Autodesk Inventor part; units mm, degrees
ref_plane "YZ Plane" through (0, 0, 0) normal (1, 0, 0) x (0, 1, 0)
ref_plane "XZ Plane" through (0, 0, 0) normal (0, 1, 0) x (-1, 0, 0)
ref_plane "XY Plane" through (0, 0, 0) normal (0, 0, 1) x (1, 0, 0)
sketch "スケッチ1" plane through (0, 0, 0) normal (0, 0, 1) x (1, 0, 0)
  line L0 (-25.3, 21.7) -> (25.3, 21.7)
  line L1 (25.3, 21.7) -> (25.3, -21.7)
  line L2 (25.3, -21.7) -> (-25.3, -21.7)
  line L3 (-25.3, -21.7) -> (-25.3, 21.7)
  circle A0 centre (-22.1, 18.5) radius 1.3
  circle A1 centre (22.1, 18.5) radius 1.3
  circle A2 centre (22.1, -18.5) radius 1.3
  circle A3 centre (-22.1, -18.5) radius 1.3
  line L4 (-18.1, 19.2) -> (-18.1, 14.5)
  line L5 (-18.1, 14.5) -> (-22.8, 14.5)
  line L6 (-22.8, 14.5) -> (-22.8, -14.5)
  line L7 (-22.8, -14.5) -> (-18.1, -14.5)
  line L8 (-18.1, -14.5) -> (-18.1, -19.2)
  line L9 (-18.1, -19.2) -> (18.1, -19.2)
  line L10 (18.1, -19.2) -> (18.1, -14.5)
  line L11 (18.1, -14.5) -> (22.8, -14.5)
  line L12 (22.8, -14.5) -> (22.8, 14.5)
  line L13 (22.8, 14.5) -> (18.1, 14.5)
  line L14 (18.1, 14.5) -> (18.1, 19.2)
  line L15 (18.1, 19.2) -> (-18.1, 19.2)
  point P0 (0, 0)
  point P1 (0, 21.7)
  point P2 (-25.3, 0)
  dimension "d0" = 50.6
  dimension "d1" = 43.4
  dimension "d2" = 2.6
  dimension "d3" = 44.2
  dimension "d4" = 37
  dimension "d5" = 22.1
  dimension "d6" = 18.5
  dimension "d7" = 2.5
  dimension "d8" = 2.5
  dimension "d9" = 2.5
  dimension "d10" = 2.5
  dimension "d11" = 4
  dimension "d12" = 4
  dimension "d13" = 4
  dimension "d14" = 4
  dimension "d15" = 4
extrude "押し出し1" add sketch "スケッチ1" along normal blind 6.9
sketch "スケッチ4" plane through (0, 0, 6.9) normal (0, 0, 1) x (1, 0, 0)
  line L0 (-18.1, 14.5) -> (-18.1, 19.2)
  line L1 (-18.1, 19.2) -> (18.1, 19.2)
  line L2 (-22.8, 14.5) -> (-18.1, 14.5)
  line L3 (-22.8, -14.5) -> (-22.8, 14.5)
  line L4 (-18.1, -14.5) -> (-22.8, -14.5)
  line L5 (-18.1, -19.2) -> (-18.1, -14.5)
  line L6 (18.1, -19.2) -> (-18.1, -19.2)
  line L7 (18.1, -14.5) -> (18.1, -19.2)
  line L8 (22.8, -14.5) -> (18.1, -14.5)
  line L9 (22.8, 14.5) -> (22.8, -14.5)
  line L10 (18.1, 14.5) -> (22.8, 14.5)
  line L11 (18.1, 19.2) -> (18.1, 14.5)
  point P0 (0, 0)
extrude "押し出し4" add sketch "スケッチ4" against normal blind 3
sketch "スケッチ3" plane through (0, 0, 6.9) normal (0, 0, 1) x (1, 0, 0)
  line L0 (-14.6, 19.9) -> (-3.9, 19.9) construction
  line L1 (-3.9, 19.9) -> (-3.9, 13.6) construction
  line L2 (-3.9, 13.6) -> (-14.6, 13.6) construction
  line L3 (-14.6, 13.6) -> (-14.6, 19.9) construction
  line L4 (-1.6, 19.9) -> (9.1, 19.9) construction
  line L5 (9.1, 19.9) -> (9.1, 13.6) construction
  line L6 (9.1, 13.6) -> (-1.6, 13.6) construction
  line L7 (-1.6, 13.6) -> (-1.6, 19.9) construction
  line L8 (13, 19.8) -> (19.3, 19.8) construction
  line L9 (19.3, 19.8) -> (19.3, 9.1) construction
  line L10 (19.3, 9.1) -> (13, 9.1) construction
  line L11 (13, 9.1) -> (13, 19.8) construction
  line L12 (25.3, 21.7) -> (-25.3, 21.7) construction
  line L13 (25.3, -21.7) -> (25.3, 21.7) construction
  line L14 (-14.8, 13.4) -> (-3.7, 13.4)
  line L15 (-3.7, 13.4) -> (-3.7, 20.1)
  line L16 (-3.7, 20.1) -> (-14.8, 20.1)
  line L17 (-14.8, 20.1) -> (-14.8, 13.4)
  line L18 (-1.8, 13.4) -> (9.3, 13.4)
  line L19 (9.3, 13.4) -> (9.3, 20.1)
  line L20 (9.3, 20.1) -> (-1.8, 20.1)
  line L21 (-1.8, 20.1) -> (-1.8, 13.4)
  line L22 (12.8, 8.9) -> (19.5, 8.9)
  line L23 (19.5, 8.9) -> (19.5, 20)
  line L24 (19.5, 20) -> (12.8, 20)
  line L25 (12.8, 20) -> (12.8, 8.9)
  point P0 (0, 0)
  dimension "d20" = 6.3
  dimension "d21" = 10.7
  dimension "d23" = 6
  dimension "d24" = 1.8
  dimension "d25" = 26.9
  dimension "d26" = 39.9
  dimension "d27" = 12.6
  dimension "d28" = 0.2
  dimension "d29" = 0.2
  dimension "d30" = 0.2
extrude "押し出し3" cut sketch "スケッチ3" along normal through all both and the other way through all
sketch "スケッチ5" plane through (0, 0, 6.9) normal (0, 0, 1) x (1, 0, 0)
  line L0 (-21.5, 13.3) -> (-13.8, 13.3) construction
  line L1 (-13.8, 13.3) -> (-13.8, 3.3) construction
  line L2 (-13.8, 3.3) -> (-21.5, 3.3) construction
  line L3 (-21.5, 3.3) -> (-21.5, 13.3) construction
  line L4 (25.3, 21.7) -> (-25.3, 21.7) construction
  line L5 (25.3, -21.7) -> (25.3, 21.7) construction
  line L6 (-25.3, 13.5) -> (-13.6, 13.5)
  line L7 (-13.6, 13.5) -> (-13.6, 3.1)
  line L8 (-13.6, 3.1) -> (-25.3, 3.1)
  line L9 (-25.3, 3.1) -> (-25.3, 13.5)
  line L10 (-25.3, 21.7) -> (-25.3, -21.7) construction
  point P0 (0, 0)
  dimension "d35" = 46.8
  dimension "d36" = 7.7
  dimension "d37" = 18.4
  dimension "d38" = 10
  dimension "d39" = 0.2
  dimension "d40" = 0.2
  dimension "d41" = 0.2
extrude "押し出し5" cut sketch "スケッチ5" against normal through all
sketch "スケッチ6" plane through (0, 0, 6.9) normal (0, 0, 1) x (1, 0, 0)
  line L0 (-5.2, 2.3) -> (-15, 2.3) construction
  line L1 (-15, 2.3) -> (-15, -11.9) construction
  line L2 (-15, -11.9) -> (-5.2, -11.9) construction
  line L3 (-5.2, -11.9) -> (-5.2, 2.3) construction
  line L4 (25.3, 21.7) -> (-25.3, 21.7) construction
  line L5 (25.3, -21.7) -> (25.3, 21.7) construction
  line L6 (-15.2, 2.5) -> (-5, 2.5)
  line L7 (-5, 2.5) -> (-5, -12.1)
  line L8 (-5, -12.1) -> (-15.2, -12.1)
  line L9 (-15.2, -12.1) -> (-15.2, 2.5)
  point P0 (0, 0)
  dimension "d44" = 14.2
  dimension "d45" = 9.8
  dimension "d46" = 40.3
  dimension "d47" = 33.6
  dimension "d48" = 0.2
extrude "押し出し6" cut sketch "スケッチ6" against normal through all
sketch "スケッチ7" plane through (0, 0, 6.9) normal (0, 0, 1) x (1, 0, 0)
  line L0 (25.3, 21.7) -> (-25.3, 21.7) construction
  line L1 (25.3, -21.7) -> (25.3, 21.7) construction
  line L2 (12.8, -5.3) -> (18.6, -5.3) construction
  line L3 (18.6, -5.3) -> (18.6, -12.8) construction
  line L4 (18.6, -12.8) -> (12.8, -12.8) construction
  line L5 (12.8, -12.8) -> (12.8, -5.3) construction
  line L6 (-9.5, -14.8) -> (-2, -14.8) construction
  line L7 (-2, -14.8) -> (-2, -20.6) construction
  line L8 (-2, -20.6) -> (-9.5, -20.6) construction
  line L9 (-9.5, -20.6) -> (-9.5, -14.8) construction
  line L10 (12.6, -13) -> (18.8, -13)
  line L11 (18.8, -13) -> (18.8, -5.1)
  line L12 (18.8, -5.1) -> (12.6, -5.1)
  line L13 (12.6, -5.1) -> (12.6, -13)
  line L14 (-1.8, -20.8) -> (-1.8, -14.6)
  line L15 (-1.8, -14.6) -> (-9.7, -14.6)
  line L16 (-9.7, -14.6) -> (-9.7, -20.8)
  line L17 (-9.7, -20.8) -> (-1.8, -20.8)
  point P0 (0, 0)
  dimension "d51" = 7.5
  dimension "d52" = 5.8
  dimension "d53" = 12.5
  dimension "d54" = 34.5
  dimension "d55" = 42.3
  dimension "d56" = 34.8
  dimension "d57" = 0.2
  dimension "d58" = 0.2
extrude "押し出し7" cut sketch "スケッチ7" against normal through all
sketch "スケッチ8" plane through (0, 0, 6.9) normal (0, 0, 1) x (1, 0, 0)
  circle A0 centre (-18, -0.6) radius 2.5 construction
  circle A1 centre (-12.5, -14.6) radius 2.5 construction
  line L0 (25.3, 21.7) -> (-25.3, 21.7) construction
  line L1 (25.3, -21.7) -> (25.3, 21.7) construction
  circle A2 centre (-18, -0.6) radius 2.7
  circle A3 centre (-12.5, -14.6) radius 2.7
  point P0 (0, 0)
  dimension "d61" = 5
  dimension "d62" = 22.3
  dimension "d63" = 36.3
  dimension "d64" = 43.3
  dimension "d65" = 37.8
  dimension "d66" = 0.2
  dimension "d67" = 0.2
extrude "押し出し8" cut sketch "スケッチ8" against normal through all
sketch "スケッチ9" plane through (0, 0, 6.9) normal (0, 0, 1) x (1, 0, 0)
  line L0 (11.3, 1.5) -> (11.3, 7.3) construction
  line L1 (11.3, 7.3) -> (17.8, 7.3) construction
  line L2 (17.8, 7.3) -> (17.8, 1.5) construction
  line L3 (17.8, 1.5) -> (16.3, 0) construction
  line L4 (16.3, 0) -> (12.8, 0) construction
  line L5 (12.8, 0) -> (11.3, 1.5) construction
  line L6 (-0.7, 1.5) -> (-0.7, 7.3) construction
  line L7 (-0.7, 7.3) -> (5.8, 7.3) construction
  line L8 (5.8, 7.3) -> (5.8, 1.5) construction
  line L9 (5.8, 1.5) -> (4.3, 0) construction
  line L10 (4.3, 0) -> (0.8, 0) construction
  line L11 (0.8, 0) -> (-0.7, 1.5) construction
  line L12 (25.3, -21.7) -> (25.3, 21.7) construction
  line L13 (25.3, 21.7) -> (-25.3, 21.7) construction
  line L14 (6, 7.5) -> (-0.9, 7.5)
  line L15 (-0.9, 7.5) -> (-0.9, 1.4172)
  line L16 (-0.9, 1.4172) -> (0.7172, -0.2)
  line L17 (0.7172, -0.2) -> (4.3828, -0.2)
  line L18 (4.3828, -0.2) -> (6, 1.4172)
  line L19 (6, 1.4172) -> (6, 7.5)
  line L20 (18, 7.5) -> (11.1, 7.5)
  line L21 (11.1, 7.5) -> (11.1, 1.4172)
  line L22 (11.1, 1.4172) -> (12.7172, -0.2)
  line L23 (12.7172, -0.2) -> (16.3828, -0.2)
  line L24 (16.3828, -0.2) -> (18, 1.4172)
  line L25 (18, 1.4172) -> (18, 7.5)
  point P0 (0, 0)
  dimension "d70" = 135
  dimension "d71" = 135
  dimension "d72" = 135
  dimension "d73" = 135
  dimension "d74" = 7.3
  dimension "d75" = 6.5
  dimension "d76" = 1.5
  dimension "d77" = 26
  dimension "d78" = 14
  dimension "d79" = 21.7
  dimension "d80" = 0.2
  dimension "d81" = 0.2
extrude "押し出し9" cut sketch "スケッチ9" against normal through all
sketch "スケッチ10" plane through (0, 0, 6.9) normal (0, 0, 1) x (1, 0, 0)
  arc A0 (-13.5198, -12.1) -> (-11.4802, -12.1) centre (-12.5, -14.6) ccw construction
  circle A1 centre (-18, -0.6) radius 2.7 construction
  line L0 (-13.6, 13.4) -> (-13.6, 3.1) construction
  line L1 (-15.2, -12.1) -> (-15.2, 2.5) construction
  line L2 (-9.7, -14.6) -> (-1.8, -14.6) construction
  line L3 (-12.5, -14.6) -> (-15.2, -14.6) construction
  line L4 (-5, -14.6881) -> (-5, -8.3419)
  line L5 (-5, -8.3419) -> (-15.2, -8.3419)
  line L6 (-15.2, -8.3419) -> (-15.2, -14.6)
  line L7 (-15.2, -14.6) -> (-12.5, -14.6)
  line L8 (-12.5, -14.6) -> (-12.5, -17.3)
  line L9 (-12.5, -17.3) -> (-5, -17.3)
  line L10 (-5, -17.3) -> (-5, -14.6881)
  line L11 (-9.7, -20.8) -> (-9.7, -14.6) construction
  line L12 (-20.7, 3.1) -> (-20.7, -0.6)
  line L13 (-20.7, -0.6) -> (-18, -0.6)
  line L14 (-18, -0.6) -> (-18, -3.3)
  line L15 (-18, -3.3) -> (-13.6, -3.3)
  line L16 (-13.6, -3.3) -> (-13.6, 3.1)
  line L17 (-13.6, 3.1) -> (-20.7, 3.1)
  point P0 (0, 0)
  point P1 (-5, -12.1)
extrude "押し出し10" cut sketch "スケッチ10" against normal through all
sketch "スケッチ11" plane through (-25.3, 21.7, 0) normal (0, 1, 0) x (1, 0, 0)
  line L0 (50.6, -6.9) -> (0, -6.9)
  line L1 (50.6, 0) -> (50.6, -6.9)
  line L2 (50.6, 0) -> (0, 0)
  line L3 (0, 0) -> (0, -6.9)
  point P0 (25.3, 0)
extrude "押し出し11" add sketch "スケッチ11" along normal blind 3.6
sketch "スケッチ12" plane through (-25.3, -21.7, 0) normal (0, -1, 0) x (1, 0, 0)
  line L0 (0, 0) -> (0, 6.9)
  line L1 (0, 0) -> (50.6, 0)
  line L2 (0, 6.9) -> (50.6, 6.9)
  line L3 (50.6, 0) -> (50.6, 6.9)
  point P0 (25.3, 0)
extrude "押し出し12" add sketch "スケッチ12" along normal blind 3.6
sketch "スケッチ13" plane through (0, 0, 0) normal (0, 0, -1) x (-1, 0, 0)
  line L0 (-25.3, 25.3) -> (25.3, 25.3)
  line L1 (25.3, -25.3) -> (-25.3, -25.3)
  line L2 (-25.3, 21.9) -> (25.3, 21.9)
  line L3 (25.3, -21.9) -> (-25.3, -21.9)
  line L4 (25.3, 21.9) -> (25.3, 25.3)
  line L5 (-25.3, 25.3) -> (-25.3, 21.9)
  line L6 (25.3, -21.9) -> (25.3, -25.3)
  line L7 (-25.3, -21.9) -> (-25.3, -25.3)
  point P0 (0, 0)
  dimension "d90" = 3.4
  dimension "d91" = 3.4
extrude "押し出し13" add sketch "スケッチ13" along normal blind 1.6
equation "\"d8\" = d7"
equation "\"d9\" = d7"
equation "\"d10\" = d7"
equation "\"d12\" = d11"
equation "\"d13\" = d11"
equation "\"d14\" = d11"
equation "\"d15\" = d11"
equation "\"d40\" = d39"
equation "\"d41\" = d39"
equation "\"d71\" = d70"
equation "\"d73\" = d72"
equation "\"d81\" = d80"
properties part number "fan_controller_case_top"
Read the model definition and answer for the solid it produces. Units are mm, in the model's axes. A direction names the side the tool comes from. Round coordinates to 2 decimals unless told otherwise and drop trailing zeros. Write each loop counter-clockwise with the first axis right and the second up, starting at its lowest first coordinate (ties: lowest second). Pieces come first, ordered by that corner, then holes. Notation, with made-up numbers: M -9.75,82 L 4.25,82 A8 ccw 4.25,87 Z; hole C 35,44 d3. An arc over 180 degrees is marked long. Use a Markdown table: item, result.
1) The part is cut by section D-D (x = 22.1). Write down the section's boundary in (y, z).
Answers follow:
| item | result |
|---|---|
| outline | M -25.3,-1.6 L -21.9,-1.6 L -21.9,0 L -19.8,0 L -19.8,6.9 L -25.3,6.9 Z; M -17.2,0 L -14.5,0 L -14.5,3.9 L 14.5,3.9 L 14.5,0 L 17.2,0 L 17.2,6.9 L -17.2,6.9 Z; M 19.8,0 L 21.9,0 L 21.9,-1.6 L 25.3,-1.6 L 25.3,6.9 L 19.8,6.9 Z |
2) A tool of negligible diameter and unlimited length cuts with its end or side. For faces 1 (the flat face through (0, -21.9, -1)), 2 (the flat face through (0, 0, 6.9)), 3 (the flat face through (-15.2, -9, 5)), 4 (the flat face through (22.8, 0, 2)), from which of +Z, -Z, +X, -X, +Y, -Y can it reach the whole face along a straight path? Write none if from no direction.
Answers follow:
| item | result |
|---|---|
| face 1 | -Z, +X, -X |
| face 2 | +Z, +X, -X, +Y, -Y |
| face 3 | +Z, -Z |
| face 4 | -Z |
3) Flat-ended cylindrical pins translate along their axes: pin 1 (6 mm diameter, centred on x = 3.5, y = 3.5, fed in from +Z); pin 2 (6 mm diameter, centred on x = -10.5, y = 6.5, fed in from -Z); pin 3 (3.5 mm diameter, centred on y = 8.5, z = 6, fed in from -X); pin 4 (14.5 mm diameter, centred on x = -16, y = -9, fed in from -Z). Find the tip coordinate at first contact, or state that the pin passes through.
Answers follow:
| item | result |
|---|---|
| pin 1 | stops at z = 6.9 |
| pin 2 | stops at z = 3.9 |
| pin 3 | stops at x = -13.6 |
| pin 4 | stops at z = 0 |
4) Straight lines are drawn through the part: line 1 along X through (y, z) = (6, 4); line 2 along Y through (x, z) = (-22.1, 4.25); line 3 along Y through (x, z) = (22.1, 5.25). For each, find the intervals that lie inside material, in ascending order. Write a range as [from, to].
Answers follow:
| item | result |
|---|---|
| line 1 | x = [-13.6, -0.9], [6, 11.1], [18, 25.3] |
| line 2 | y = [-25.3, -19.8], [-17.2, 3.1], [13.5, 17.2], [19.8, 25.3] |
| line 3 | y = [-25.3, -19.8], [-17.2, 17.2], [19.8, 25.3] |
5) The part is cut by section B-B (y = -18.5). Write down the section's boundary in (x, z), plus the area to 3 significant figures.
Answers follow:
| item | result |
|---|---|
| outline | M -25.3,0 L -23.4,0 L -23.4,6.9 L -25.3,6.9 Z; M -20.8,0 L -18.1,0 L -18.1,3.9 L -9.7,3.9 L -9.7,6.9 L -20.8,6.9 Z; M -1.8,3.9 L 18.1,3.9 L 18.1,0 L 20.8,0 L 20.8,6.9 L -1.8,6.9 Z; M 23.4,0 L 25.3,0 L 25.3,6.9 L 23.4,6.9 Z |
| area | 148 mm2 |
6) For a pull along X with two mould halves and no side action, classify faces 5 (the flat face through (3, 7.5, 5)), 6 (the flat face through (-0.1, -19.4, 0)), 7 (the flat face through (-25.3, -11, 4)) as pulls with the +X half, pulls with the -X half, needs draft (parallel to the pull), parting line crosses it, or undercut.
Answers follow:
| item | result |
|---|---|
| face 5 | undercut |
| face 6 | needs draft |
| face 7 | pulls with the -X half |
7) The part is cut by section C-C (y = 18.5). Write down the section's boundary in (x, z).
Answers follow:
| item | result |
|---|---|
| outline | M -25.3,0 L -23.4,0 L -23.4,6.9 L -25.3,6.9 Z; M -20.8,0 L -18.1,0 L -18.1,3.9 L -14.8,3.9 L -14.8,6.9 L -20.8,6.9 Z; M -3.7,3.9 L -1.8,3.9 L -1.8,6.9 L -3.7,6.9 Z; M 9.3,3.9 L 12.8,3.9 L 12.8,6.9 L 9.3,6.9 Z; M 19.5,0 L 20.8,0 L 20.8,6.9 L 19.5,6.9 Z; M 23.4,0 L 25.3,0 L 25.3,6.9 L 23.4,6.9 Z |
8) The part is cut by section A-A (x = -22.1). Write down the section's boundary in (y, z).
Answers follow:
| item | result |
|---|---|
| outline | M -25.3,-1.6 L -21.9,-1.6 L -21.9,0 L -19.8,0 L -19.8,6.9 L -25.3,6.9 Z; M -17.2,0 L -14.5,0 L -14.5,3.9 L 3.1,3.9 L 3.1,6.9 L -17.2,6.9 Z; M 13.5,3.9 L 14.5,3.9 L 14.5,0 L 17.2,0 L 17.2,6.9 L 13.5,6.9 Z; M 19.8,0 L 21.9,0 L 21.9,-1.6 L 25.3,-1.6 L 25.3,6.9 L 19.8,6.9 Z |
